```python
from build123d import *

# Parameters (mm, degrees)
SKETCH21_R              = 5
CUT_EXTRUDE3_DEPTH      = 10.5
CUT_EXTRUDE3_DEPTH_BACK = 210.883244548


with BuildPart() as part:
    # Sweep-Thin3: sweep along a curve in space
    with BuildLine() as sweep_thin3_path:
        Line((0, 0, 0), (150, 0, 0))
        Line((150, 0, 0), (363.169892788, -200, 500))
        Line((363.169892788, -200, 500), (363.169892788, -200, 530))
    # Sketch2 → Sweep-Thin3 (sweep)
    with BuildSketch(Plane(origin=(0, 0, 0), x_dir=(0, 0, -1), z_dir=(1, 0, 0))):
        with BuildLine():
            Line((1.5, 9.5), (-1.5, 9.5))
            ThreePointArc((-1.5, 9.5), (-7.156854249, 7.156854249), (-9.5, 1.5))
            Line((-9.5, 1.5), (-9.5, -1.5))
            ThreePointArc((-9.5, -1.5), (-7.156854249, -7.156854249), (-1.5, -9.5))
            Line((-1.5, -9.5), (1.5, -9.5))
            ThreePointArc((1.5, -9.5), (7.156854249, -7.156854249), (9.5, -1.5))
            Line((9.5, -1.5), (9.5, 1.5))
            ThreePointArc((9.5, 1.5), (7.156854249, 7.156854249), (1.5, 9.5))
        make_face()
        with BuildLine():
            Line((1.5, 6.5), (-1.5, 6.5))
            ThreePointArc((-1.5, 6.5), (-5.035533906, 5.035533906), (-6.5, 1.5))
            Line((-6.5, 1.5), (-6.5, -1.5))
            ThreePointArc((-6.5, -1.5), (-5.035533906, -5.035533906), (-1.5, -6.5))
            Line((-1.5, -6.5), (1.5, -6.5))
            ThreePointArc((1.5, -6.5), (5.035533906, -5.035533906), (6.5, -1.5))
            Line((6.5, -1.5), (6.5, 1.5))
            ThreePointArc((6.5, 1.5), (5.035533906, 5.035533906), (1.5, 6.5))
        make_face(mode=Mode.SUBTRACT)
    sweep(path=sweep_thin3_path.line, transition=Transition.RIGHT)

    # Sketch21 → Cut-Extrude3 (cut, two sides)
    with BuildSketch(Plane(origin=(0, 0, 0), x_dir=(1, 0, 0), z_dir=(0, 1, 0))) as cut_extrude3_sk:
        with Locations((50, 0)):
            Circle(SKETCH21_R)
    extrude(amount=CUT_EXTRUDE3_DEPTH, mode=Mode.SUBTRACT)
    extrude(cut_extrude3_sk.sketch, amount=-CUT_EXTRUDE3_DEPTH_BACK, mode=Mode.SUBTRACT)


solid = part.part
```
Work out the finished part from the listing and answer in its coordinate system (mm). A direction names the side the tool comes from. Give positions to 0.01 mm unless a question says otherwise; leave off trailing zeros. Loops run counter-clockwise (first coordinate to the right, second up) from the corner with the lowest first, then second, coordinate; pieces in that order, holes last. Notation, with made-up numbers: (5, -2.5) -> (15, -2.5) arc R14 ccw to (15, 13.5) -> close; hole circle Ø4 at (-39, 50.5). An arc over 180 degrees is marked (long way). Put each result on its own line as item: value. Start each with the question number.
Item 1: Which of the six approach directions +Z, -Z, +X, -X, +Y, -Y give full straight-line access (tool end or side, diameter ignored) to faces 4 (the face through (259.76, -94.95, 253.65)), 5 (the face through (261.2, -109.05, 247.49))?
Item 2: Find the intervals of material crossed by L1, parallel to Z at x = 50, y = -6.95; L2, parallel to X at y = -141, z = 357; L3, parallel to Z at x = 50, y = 7.4, in increasing order. Write a range as [from, to].
Item 3: The part is cut by section A-A (x = 120). Give the vertices of the cut face in (y, z).
Item 4: Each of these flat-tipped pins is pushed along its axis until it touches: P1, Ø2.5, axis at x = 116, z = 0, coming from the -Y side; P2, Ø0.9, axis at x = 100.5, y = 0.5, coming from the +Z side; P3, Ø10, axis at y = -127, z = 345, coming from the +X side. Where does it stop, or does it pass through?
Item 5: The mould has two halves that part along Y. Classify faces 1 (the face through (265.58, -102.84, 247.55)), 2 (the face through (255.18, -95.364, 256.092)), 3 (the face through (253.91, -92.76, 257.04)): released by +Y, released by -Y, zero draft, split by the parting line, or undercut.
Answers below:
1. face 4: none
1. face 5: -Z, -Y
2. L1: [-7.36, -5], [5, 7.36]
2. L2: [291.67, 295.13], [309.34, 312.59]
2. L3: [-6.9, -5], [5, 6.9]
3. outline: (-9.5, -1.5) arc R8 ccw to (-1.5, -9.5) -> (1.5, -9.5) arc R8 ccw to (9.5, -1.5) -> (9.5, 1.5) arc R8 ccw to (1.5, 9.5) -> (-1.5, 9.5) arc R8 ccw to (-9.5, 1.5) -> close; hole (-6.5, -1.5) arc R5 ccw to (-1.5, -6.5) -> (1.5, -6.5) arc R5 ccw to (6.5, -1.5) -> (6.5, 1.5) arc R5 ccw to (1.5, 6.5) -> (-1.5, 6.5) arc R5 ccw to (-6.5, 1.5) -> close
4. P1: y = -9.5
4. P2: z = 9.5
4. P3: x = 305.25
5. face 1: released by -Y
5. face 2: undercut
5. face 3: released by +Y
